Check sheet for the modelled part. Datum: model origin and axes. Units: mm. Round coordinates to 2 decimals unless told otherwise and drop trailing zeros. Write each loop counter-clockwise with the first axis right and the second up, starting at its lowest first coordinate (ties: lowest second). Pieces come first, ordered by that corner, then holes.
Item 1: Material ranges on line 1 (X direction, y = 6.5, z = -24.5); line 2 (X direction, y = 1.25, z = -29.5); line 3 (Z direction, x = 62.5, y = 5.75), recorded low to high.
Item 2: Cross-section at C-C on x = 7. Enter the section's corners in (y, z).
Item 3: Release check for a two-part mould opening along Z. For faces 1 (the flat face through (98, 7, -25)), 2 (the cylindrical face through (57.138, 2.535, -28.11)), 3 (the flat face through (49, 8, -3)) record: +Z half, -Z half, draft (parallel to the pull), parting line (faces both ways), or undercut.
Item 4: Cross-section at D-D on y = 2.5. Enter the section's corners in (x, z).
Item 5: Cross-section at A-A on y = 7.75. Enter the section's corners in (x, z).
Item 6: Cross-section at B-B on z = -19.5. Count the separate pieces of the cut face and the enclosed holes in it, plus the area to 3 significant figures.
Item 7: Go/stop test with flat-tipped pins: pin 1 Ø12 at (x, z) = (28, -24) entering from -Y; pin 2 Ø9.5 at (x, z) = (24.73, -24.54) entering from -Y. Record where each tip stops, or that it passes through.
from build123d import *

# Parameters (mm, degrees)
SKIZZE1_W                       = 100
SKIZZE1_H                       = 50
AUFSATZ_LINEAR_AUSTRAGEN1_DEPTH = 10
SKIZZE2_R                       = 5.979005814
SCHNITT_LINEAR_AUSTRAGEN1_DEPTH = 11
FASE1_SIZE                      = 5
SKIZZE3_R                       = 8.504790413
SCHNITT_MIT_EXTRA_FASE_DEPTH    = 11
FASE2_SIZE                      = 5


with BuildPart() as part:
    # Skizze1 → Aufsatz-Linear austragen1 (new body)
    with BuildSketch(Plane(origin=(0, 0, 0), x_dir=(1, 0, 0), z_dir=(0, 1, 0))):
        with Locations((50, 25)):
            Rectangle(SKIZZE1_W, SKIZZE1_H)
    extrude(amount=AUFSATZ_LINEAR_AUSTRAGEN1_DEPTH)

    # Skizze2 → Schnitt-Linear austragen1 (cut, through all)
    with BuildSketch(Plane(origin=(0, 10, 0), x_dir=(1, 0, 0), z_dir=(0, 1, 0))):
        with Locations(Location((24.734846156, 24.536515152, 0), (0, 0, 270))):  # turned: the seam where the file's is
            Circle(SKIZZE2_R)
    extrude(amount=-SCHNITT_LINEAR_AUSTRAGEN1_DEPTH, mode=Mode.SUBTRACT)

    # Fase1
    fase1_edges = [part.edges().sort_by_distance(p)[0] for p in [
        (100, 10, -25),
        (24.734846156, 10, -30.515520966),
        (50, 10, 0),
    ]]
    chamfer(fase1_edges, length=FASE1_SIZE)

    # Skizze3 → Schnitt mit extra Fase (cut, through all)
    with BuildSketch(Plane(origin=(0, 10, 0), x_dir=(1, 0, 0), z_dir=(0, 1, 0))):
        with Locations(Location((65.440217499, 26.266772753, 0), (0, 0, 270))):  # turned: the seam where the file's is
            Circle(SKIZZE3_R)
    extrude(amount=-SCHNITT_MIT_EXTRA_FASE_DEPTH, mode=Mode.SUBTRACT)

    # Fase2
    fase2_edges = [part.edges().sort_by_distance(p)[0] for p in [
        (65.440217499, 10, -34.771563166),
    ]]
    chamfer(fase2_edges, length=FASE2_SIZE)


solid = part.part
Response values:
1. line 1: x = 0 to 17.26, 32.21 to 55.59, 75.29 to 98.5
1. line 2: x = 0 to 21.4, 28.07 to 57.57, 73.31 to 100
1. line 3: z = -50 to -35.04, -17.49 to -0.75
2. outline: (0, -50) - (10, -50) - (10, -5) - (5, 0) - (0, 0) - close
3. face 1: draft
3. face 2: undercut
3. face 3: +Z half
4. outline: (0, -50) - (100, -50) - (100, 0) - (0, 0) - close; hole circle Ø11.96 at (24.73, -24.54); hole circle Ø17.01 at (65.44, -26.27)
5. outline: (0, -50) - (97.25, -50) - (97.25, -2.75) - (0, -2.75) - close; hole circle Ø17.46 at (24.73, -24.54); hole circle Ø22.51 at (65.44, -26.27)
6. separate pieces: 3
6. enclosed holes: 0
6. area: 751 mm2
7. pin 1: stops at y = 0
7. pin 2: passes through
